Geometry: final body of the model. Coordinates: model frame, mm. A direction names the side the tool comes from. Give positions to 0.01 mm unless a question says otherwise; leave off trailing zeros. Write each loop counter-clockwise with the first axis right and the second up, starting at its lowest first coordinate (ties: lowest second). Pieces come first, ordered by that corner, then holes. Notation, with made-up numbers: M -38.75,-39.5 L 9.25,-39.5 A20 cw 9.25,-21.5 Z; hole C 72,-20.75 d4. An arc over 180 degrees is marked long. One line per question, with ' | ' between items.
from build123d import *

# Parameters (mm, degrees)
F0_W          = 300
F0_H          = 500
F1_DEPTH      = 100
F4_DEPTH      = 225
F4_DEPTH_BACK = 225
F5_DEPTH      = 225
F5_DEPTH_BACK = 225
F2_R          = 7.5
F6_DEPTH      = 25
F7_R          = 6
F8_DEPTH      = 25
F9_R          = 6
F10_DEPTH     = 25
F11_R         = 3
F12_DEPTH     = 10
F13_R         = 3
F14_DEPTH     = 10
F15_R         = 5
F16_DEPTH     = 15


# Not quite as in the source:
# - a feature of the source that left no trace in its solid (it failed there, or was rolled back) is left out


with BuildPart() as f1:
    # F0 (on Top) → F1 (new body)
    with BuildSketch(Plane.XY):
        Rectangle(F0_W, F0_H)
    extrude(amount=F1_DEPTH)

    # F3 (on Front) → F4 (cut, two sides)
    with BuildSketch(Plane.XZ) as f4_sk:
        Polygon((150, 17.5), (150, 82.5), (120, 82.5), (120, 67.5), (140, 67.5), (140, 32.5), (120, 32.5), (120, 17.5), align=None)
        Polygon((-120, 82.5), (-150, 82.5), (-150, 17.5), (-120, 17.5), (-120, 32.5), (-140, 32.5), (-140, 67.5), (-120, 67.5), align=None)
    extrude(amount=-F4_DEPTH, mode=Mode.SUBTRACT)
    extrude(f4_sk.sketch, amount=F4_DEPTH_BACK, mode=Mode.SUBTRACT)

    # F3 (on Front) → F5 (join, two sides)
    with BuildSketch(Plane.XZ) as f5_sk:
        Polygon((150, 17.5), (150, 82.5), (120, 82.5), (120, 67.5), (140, 67.5), (140, 32.5), (120, 32.5), (120, 17.5), align=None)
        Polygon((-120, 82.5), (-150, 82.5), (-150, 17.5), (-120, 17.5), (-120, 32.5), (-140, 32.5), (-140, 67.5), (-120, 67.5), align=None)
    extrude(amount=F5_DEPTH)
    extrude(f5_sk.sketch, amount=-F5_DEPTH_BACK)

    # F2 (on face) → F6 (cut)
    with BuildSketch(Plane(origin=(0, 0, 0), x_dir=(1, 0, 0), z_dir=(0, 0, -1))):
        with Locations((-100, 200)):
            Circle(F2_R)
        with Locations((100, 200)):
            Circle(F2_R)
        with Locations((100, -200)):
            Circle(F2_R)
        with Locations((-100, -200)):
            Circle(F2_R)
    extrude(amount=-F6_DEPTH, mode=Mode.SUBTRACT)

    # F7 (on face) → F8 (cut)
    with BuildSketch(Plane(origin=(-150, 0, 0), x_dir=(0, -1, 0), z_dir=(-1, 0, 0))):
        with Locations((-178.5714285714, 50)):
            Circle(F7_R)
        with Locations((-107.1428571429, 50)):
            Circle(F7_R)
        with Locations((-35.7142857143, 50)):
            Circle(F7_R)
        with Locations((35.7142857143, 50)):
            Circle(F7_R)
        with Locations((107.1428571429, 50)):
            Circle(F7_R)
        with Locations((178.5714285714, 50)):
            Circle(F7_R)
    extrude(amount=-F8_DEPTH, mode=Mode.SUBTRACT)

    # F9 (on face) → F10 (cut)
    with BuildSketch(Plane.YZ.offset(150)):
        with Locations((-178.5714285714, 50)):
            Circle(F9_R)
        with Locations((-107.1428571429, 50)):
            Circle(F9_R)
        with Locations((-35.7142857143, 50)):
            Circle(F9_R)
        with Locations((35.7142857143, 50)):
            Circle(F9_R)
        with Locations((107.1428571429, 50)):
            Circle(F9_R)
        with Locations((178.5714285714, 50)):
            Circle(F9_R)
    extrude(amount=-F10_DEPTH, mode=Mode.SUBTRACT)

    # F11 (on face) → F12 (cut)
    with BuildSketch(Plane(origin=(0, 250, 0), x_dir=(-1, 0, 0), z_dir=(0, 1, 0))):
        with Locations((-135, 85)):
            Circle(F11_R)
        with Locations((-135, 15)):
            Circle(F11_R)
        with Locations((135, 15)):
            Circle(F11_R)
        with Locations((135, 85)):
            Circle(F11_R)
    extrude(amount=-F12_DEPTH, mode=Mode.SUBTRACT)

    # F13 (on face) → F14 (cut)
    with BuildSketch(Plane.XZ.offset(250)):
        with Locations((135, 85)):
            Circle(F13_R)
        with Locations((135, 15)):
            Circle(F13_R)
        with Locations((-135, 15)):
            Circle(F13_R)
        with Locations((-135, 85)):
            Circle(F13_R)
    extrude(amount=-F14_DEPTH, mode=Mode.SUBTRACT)

    # F15 (on face) → F16 (cut)
    with BuildSketch(Plane.XY.offset(100)):
        with Locations((120, 220)):
            Circle(F15_R)
        with Locations((120, 132)):
            Circle(F15_R)
        with Locations((120, 44)):
            Circle(F15_R)
        with Locations((120, -44)):
            Circle(F15_R)
        with Locations((120, -132)):
            Circle(F15_R)
        with Locations((120, -220)):
            Circle(F15_R)
        with Locations((40, 220)):
            Circle(F15_R)
        with Locations((40, 132)):
            Circle(F15_R)
        with Locations((40, 44)):
            Circle(F15_R)
        with Locations((40, -44)):
            Circle(F15_R)
        with Locations((40, -132)):
            Circle(F15_R)
        with Locations((40, -220)):
            Circle(F15_R)
        with Locations((-40, 220)):
            Circle(F15_R)
        with Locations((-40, 132)):
            Circle(F15_R)
        with Locations((-40, 44)):
            Circle(F15_R)
        with Locations((-40, -44)):
            Circle(F15_R)
        with Locations((-40, -132)):
            Circle(F15_R)
        with Locations((-40, -220)):
            Circle(F15_R)
        with Locations((-120, 220)):
            Circle(F15_R)
        with Locations((-120, 132)):
            Circle(F15_R)
        with Locations((-120, 44)):
            Circle(F15_R)
        with Locations((-120, -44)):
            Circle(F15_R)
        with Locations((-120, -132)):
            Circle(F15_R)
        with Locations((-120, -220)):
            Circle(F15_R)
    extrude(amount=-F16_DEPTH, mode=Mode.SUBTRACT)


solid = f1.part
(1) Material intervals for L1, parallel to X at y = 197, z = 12.5, sorted ascending. Write a range as [from, to].
Working result:
L1: x = [-150, -106.87], [-93.13, 93.13], [106.87, 150]
(2) Set-up query: faces 5 (the face through (-2, -250, 49)), 6 (the face through (-40, 220, 85)), 7 (the face through (125, -36, 50)), 8 (the face through (-125, -36, 50)). Return all of +Z, -Z, +X, -X, +Y, -Y with unobstructed straight access to the full face (end or side cutting, diameter ignored); none if empty.
Working result:
face 5: +Z, -Z, +X, -X, -Y | face 6: +Z | face 7: +X | face 8: -X
(3) Cut plane B-B, the plane y = -200. Return loops of the section in (x, z), then the cut area to 4 significant figures.
Working result:
outline: M -150,0 L -107.5,0 L -107.5,25 L -92.5,25 L -92.5,0 L 92.5,0 L 92.5,25 L 107.5,25 L 107.5,0 L 150,0 L 150,100 L -150,100 Z | area: 29,250 mm^2
(4) Cut plane A-A, the plane x = -100. Return loops of the section in (y, z), then the cut area to 4 significant figures.
Working result:
outline: M -250,0 L -207.5,0 L -207.5,25 L -192.5,25 L -192.5,0 L 192.5,0 L 192.5,25 L 207.5,25 L 207.5,0 L 250,0 L 250,100 L -250,100 Z | area: 49,250 mm^2
(5) First-contact query: P1, Ø5, axis at x = 118, y = 131, coming from the +Z side; P2, Ø9.5, axis at y = -107.5, z = 51, coming from the +X side; P3, Ø14, axis at y = 35.71, z = 50, coming from the -X side; P4, Ø1.8, axis at x = -135, z = 85, coming from the -Y side. Flat tips, straight axial feed; report the tip coordinate or a pass-through.
Working result:
P1: stops at z = 85 | P2: stops at x = 125 | P3: stops at x = -150 | P4: stops at y = -240
(6) Draft query along X for faces 1 (the face through (36, 47, 93)), 2 (the face through (36, -41, 93)), 3 (the face through (125, 36, 50)), 4 (the face through (137.68, -101.42, 51.8)). Return one class per face: released by +X, released by -X, zero draft, split by the parting line, or undercut.
Working result:
face 1: undercut | face 2: undercut | face 3: released by +X | face 4: zero draft
